```python
from build123d import *

# Parameters (mm, degrees)
IZIM1_W                     = 30
IZIM1_H                     = 70
Y_KSEKLIK_EKSTR_ZYON1_DEPTH = 30
IZIM2_W                     = 40
IZIM2_H                     = 80
Y_KSEKLIK_EKSTR_ZYON2_DEPTH = 5
RADYUS1_R                   = 5
RADYUS2_R                   = 5
RADYUS3_R                   = 5
RADYUS4_R                   = 5
IZIM4_W                     = 15
IZIM4_H                     = 50
IZIM4_W_2                   = 10
KES_EKSTR_ZYON1_DEPTH       = 59
IZIM5_R                     = 20
Y_KSEKLIK_EKSTR_ZYON4_DEPTH = 30
IZIM6_W                     = 25
IZIM6_H                     = 10
KES_EKSTR_ZYON4_DEPTH       = 7
IZIM7_W                     = 25
IZIM7_H                     = 10
KES_EKSTR_ZYON6_DEPTH       = 7
Y_KSEKLIK_EKSTR_ZYON5_DEPTH = 16
IZIM13_W                    = 40
IZIM13_H                    = 5
Y_KSEKLIK_EKSTR_ZYON6_DEPTH = 60
Y_KSEKLIK_EKSTR_ZYON7_DEPTH = 5
Y_KSEKLIK_EKSTR_ZYON8_DEPTH = 5


with BuildPart() as part:
    # Çizim1 → Yükseklik-Ekstrüzyon1 (new body)
    with BuildSketch(Plane.XY):
        Polygon((5, 0), (0, 0), (0, -5), (0, -80), (35, -80), (40, -80), (40, -75), (40, -5), (40, 0), (35, 0), align=None)
        with Locations((20, -40)):
            Rectangle(IZIM1_W, IZIM1_H, mode=Mode.SUBTRACT)
    extrude(amount=Y_KSEKLIK_EKSTR_ZYON1_DEPTH)

    # Çizim2 → Yükseklik-Ekstrüzyon2 (add)
    with BuildSketch(Plane(origin=(0, 0, 0), x_dir=(-1, 0, 0), z_dir=(0, 0, -1))):
        with Locations((-20, -40)):
            Rectangle(IZIM2_W, IZIM2_H)
    extrude(amount=-Y_KSEKLIK_EKSTR_ZYON2_DEPTH)

    # Radyus1
    radyus1_edges = [part.edges().sort_by_distance(p)[0] for p in [
        (40, 0, 15),
    ]]
    fillet(radyus1_edges, radius=RADYUS1_R)

    # Radyus2
    radyus2_edges = [part.edges().sort_by_distance(p)[0] for p in [
        (0, 0, 15),
    ]]
    fillet(radyus2_edges, radius=RADYUS2_R)

    # Radyus3
    radyus3_edges = [part.edges().sort_by_distance(p)[0] for p in [
        (0, -80, 15),
    ]]
    fillet(radyus3_edges, radius=RADYUS3_R)

    # Radyus4
    radyus4_edges = [part.edges().sort_by_distance(p)[0] for p in [
        (40, -80, 15),
    ]]
    fillet(radyus4_edges, radius=RADYUS4_R)

    # Çizim4 → Kes-Ekstrüzyon1 (cut)
    with BuildSketch(Plane(origin=(40, 0, 0), x_dir=(0, 0, -1), z_dir=(1, 0, 0))):
        with Locations((-22.5, -40)):
            Rectangle(IZIM4_W, IZIM4_H)
        with Locations((-10, -40)):
            Rectangle(IZIM4_W_2, IZIM4_H)
    extrude(amount=-KES_EKSTR_ZYON1_DEPTH, mode=Mode.SUBTRACT)

    # Çizim5 → Yükseklik-Ekstrüzyon4 (add)
    with BuildSketch(Plane(origin=(0, 0, 0), x_dir=(-1, 0, 0), z_dir=(0, 0, -1))):
        with Locations((-20, -49.329631519)):
            Circle(IZIM5_R)
    extrude(amount=-Y_KSEKLIK_EKSTR_ZYON4_DEPTH)

    # Çizim6 → Kes-Ekstrüzyon4 (cut)
    with BuildSketch(Plane(origin=(40, 0, 0), x_dir=(0, 0, -1), z_dir=(1, 0, 0))):
        with Locations((-17.5, -70)):
            Rectangle(IZIM6_W, IZIM6_H)
    extrude(amount=-KES_EKSTR_ZYON4_DEPTH, mode=Mode.SUBTRACT)

    # Çizim7 → Kes-Ekstrüzyon6 (cut)
    with BuildSketch(Plane.ZY):
        with Locations((17.5, -70)):
            Rectangle(IZIM7_W, IZIM7_H)
    extrude(amount=-KES_EKSTR_ZYON6_DEPTH, mode=Mode.SUBTRACT)

    # Çizim12 → Yükseklik-Ekstrüzyon5 (add)
    with BuildSketch(Plane(origin=(0, 0, 0), x_dir=(-1, 0, 0), z_dir=(0, 0, -1))):
        Polygon((-35.259105609, -28.804442177), (-40, -28.804442177), (-40, -33.804442177), (-40, -75), (-35, -75), (-35, -33.804442177), (-5, -33.804442177), (-5, -75), (0, -75), (0, -33.804442177), (0, -28.804442177), (-5, -28.804442177), (-35, -28.804442177), align=None)
    extrude(amount=Y_KSEKLIK_EKSTR_ZYON5_DEPTH)

    # Çizim13 → Yükseklik-Ekstrüzyon6 (add)
    with BuildSketch(Plane(origin=(0, 0, -16), x_dir=(-1, 0, 0), z_dir=(0, 0, -1))):
        with Locations((-20, -31.304442177)):
            Rectangle(IZIM13_W, IZIM13_H)
    extrude(amount=Y_KSEKLIK_EKSTR_ZYON6_DEPTH)

    # Çizim14 → Yükseklik-Ekstrüzyon7 (add)
    with BuildSketch(Plane(origin=(40, 0, 0), x_dir=(0, 0, -1), z_dir=(1, 0, 0))):
        Polygon((0, -5), (38, -28.804442177), (0, -28.804442177), align=None)
    extrude(amount=-Y_KSEKLIK_EKSTR_ZYON7_DEPTH)

    # Çizim15 → Yükseklik-Ekstrüzyon8 (add)
    with BuildSketch(Plane.ZY):
        Polygon((-38, -28.804442177), (0, -5), (0, -28.804442177), align=None)
    extrude(amount=-Y_KSEKLIK_EKSTR_ZYON8_DEPTH)


solid = part.part
```
Part model, mm, in its own coordinate system. A direction names the side the tool comes from. Round coordinates to 2 decimals unless told otherwise and drop trailing zeros. Write each loop counter-clockwise with the first axis right and the second up, starting at its lowest first coordinate (ties: lowest second). Pieces come first, ordered by that corner, then holes. Notation, with made-up numbers: M -16,-14.75 L 32,-14.75 A30 ccw 32,19.25 Z; hole C -11.75,72.25 d4. An arc over 180 degrees is marked long. Answer as CSV lines item,"result". Start each with the question number.
1) Which spindle directions (+Z, -Z, +X, -X, +Y, -Y) get a long thin tool onto all of the face, cutting with end or side? Do faces 5 (the face through (3, -15, 17)), 6 (the face through (20, -5, 17)), 7 (the face through (20, -14, 0)). Say none if no direction does.
2) Band-saw the part on C-C (x = 20). List the corners of the cut face in (y, z).
3) Mould opens along Y. For faces 1 (the face through (20, -75, 18)), 2 (the face through (2, -1, 15)), 3 (the face through (0.924, -43.322, 17.325)), 4 (the face through (20, -4, 30)) say: +Y half, -Y half, draft (parallel to the pull), parting line (faces both ways), or undercut.
4) Band-saw the part on A-A (z = 18). List the corners of the cut face in (x, y), then the cut area to 3 significant figures.
5) Drill centre lines: L1, parallel to X at y = -14, z = 16; L2, parallel to Z at x = 19.5, y = -57; L3, parallel to Y at x = 10.5, z = -58. Where is each one in solid material? Low to high.
6) Band-saw the part on B-B (y = -72). List the corners of the cut face in (x, z).
7) Band-saw the part on D-D (z = -10). List the corners of the cut face in (x, y), then the cut area to 3 significant figures.
8) Drop flat-ended pins along their axis: pin 1 (3 mm diameter, centred on x = 33.5, y = -69, fed in from +Z); pin 2 (6 mm diameter, centred on y = -60, z = 16.5, fed in from -X); pin 3 (2.5 mm diameter, centred on x = 38.5, z = -4, fed in from -Y). Give the stop position or say it passes through.
Worked out:
1,face 5,"+Z, +X, -X"
1,face 6,"+Z"
1,face 7,"-Z, +Y"
2,outline,"M -80,0 L -33.8,0 L -33.8,-76 L -28.8,-76 L -28.8,0 L 0,0 L 0,30 L -5,30 L -5,5 L -29.33,5 L -29.33,30 L -69.33,30 L -69.33,5 L -75,5 L -75,30 L -80,30 Z"
3,face 1,"undercut"
3,face 2,"+Y half"
3,face 3,"undercut"
3,face 4,"draft"
4,outline,"M 0,-75 A5 ccw 5,-80 L 35,-80 A5 ccw 40,-75 Z; C 20,-49.33 d40; M 0,-15 L 5,-15 L 5,-5 L 35,-5 L 35,-15 L 40,-15 L 40,-5 A5 ccw 35,0 L 5,0 A5 ccw 0,-5 Z"
4,area,"1,740 mm²"
5,L1,"0 to 5, 35 to 40"
5,L2,"0 to 30"
5,L3,"-33.8 to -28.8"
6,outline,"M 0,-16 L 5,-16 L 5,0 L 35,0 L 35,-16 L 40,-16 L 40,5 L 0,5 Z"
7,outline,"M 0,-75 L 5,-75 L 5,-33.8 L 35,-33.8 L 35,-75 L 40,-75 L 40,-11.26 L 35,-11.26 L 35,-28.8 L 5,-28.8 L 5,-11.26 L 0,-11.26 Z"
7,area,"787 mm²"
8,pin 1,"z = 5"
8,pin 2,"x = 1.53"
8,pin 3,"y = -75"
